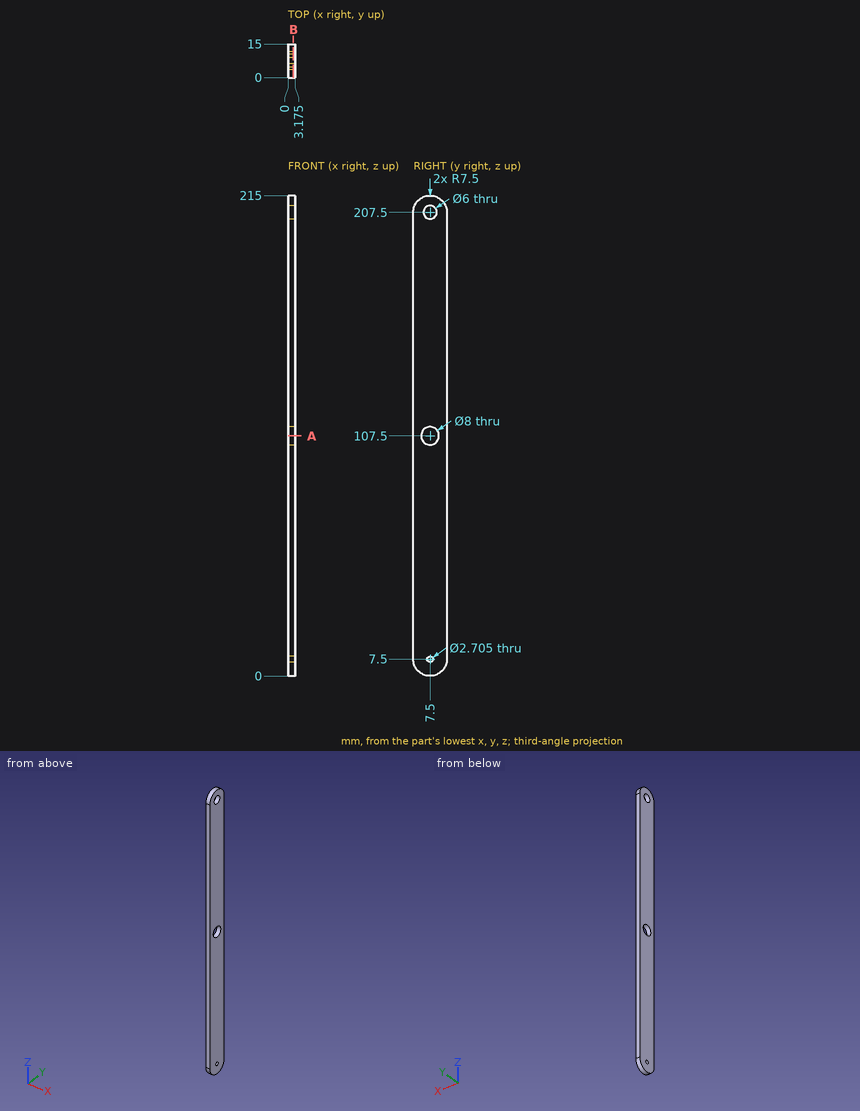
Print and shaded views of the part. All mm, measured from the part's lowest x, y and z. Coordinates: 2 decimals unless noted, no trailing zeros. Order: outer loops, then holes, each group sorted by start corner. A loop starts at its lowest first (then second) coordinate and runs counter-clockwise, first axis right, second up. Notation, with made-up numbers: (16.5, 56) -> (46.5, 56) arc R23 cw to (46.5, 67) -> close; hole circle Ø11 at (-5, 3.5). An arc over 180 degrees is marked (long way). Answer as a JSON object with one key per item and string values. Group by question number.
1) Cut at A-A, the plane z = 107.5. Write the cut outline in (x, y) (3 decimals).
2) Cut at B-B, the plane x = 2.3. Write the cut outline in (y, z) (1 decimal).
3) Drill centre lines: L1, parallel to Y at x = 0.7, z = 207.5; L2, parallel to Y at x = 2.35, z = 107.5; L3, parallel to Z at x = 3, y = 5.5. Where is each one in solid material? Low to high.
4) Flat gauge pins, fed straight in: pin 1 (1.5 mm diameter, centred on x = 1, y = 6.5, fed in from -Z); pin 2 (7 mm diameter, centred on y = 7.5, z = 107.5, fed in from +X). Where does each tip first touch, or does it go through?
Check values:
{
 "1": {"outline": "(0, 0) -> (3.175, 0) -> (3.175, 3.5) -> (0, 3.5) -> close; (0, 11.5) -> (3.175, 11.5) -> (3.175, 15) -> (0, 15) -> close"},
 "2": {"outline": "(0, 7.5) arc R7.5 ccw to (15, 7.5) -> (15, 207.5) arc R7.5 ccw to (0, 207.5) -> close; hole circle Ø8 at (7.5, 107.5); hole circle Ø6 at (7.5, 207.5); hole circle Ø2.7 at (7.5, 7.5)"},
 "3": {"L1": "y = 0 to 4.5, 10.5 to 15", "L2": "y = 0 to 3.5, 11.5 to 15", "L3": "z = 0.27 to 104.04, 110.96 to 205.26, 209.74 to 214.73"},
 "4": {"pin 1": "stops at z = 0", "pin 2": "passes through"}
}
